```python
from build123d import *

# Parameters (mm, degrees)
SKETCH1_R           = 36.83
SKETCH1_R_2         = 24.13
SKETCH1_R_3         = 2.15265
BOSS_EXTRUDE1_DEPTH = 6.35


with BuildPart() as part:
    # Sketch1 → Boss-Extrude1 (new body)
    with BuildSketch(Plane(origin=(0, 0, 0), x_dir=(1, 0, 0), z_dir=(0, 1, 0))):
        Circle(SKETCH1_R)
        Circle(SKETCH1_R_2, mode=Mode.SUBTRACT)
        with Locations((0, 30.48)):
            Circle(SKETCH1_R_3, mode=Mode.SUBTRACT)
        with Locations((11.664191018, 28.159848151)):
            Circle(SKETCH1_R_3, mode=Mode.SUBTRACT)
        with Locations((21.552614691, 21.552614691)):
            Circle(SKETCH1_R_3, mode=Mode.SUBTRACT)
        with Locations((28.159848151, 11.664191018)):
            Circle(SKETCH1_R_3, mode=Mode.SUBTRACT)
        with Locations((30.48, 0)):
            Circle(SKETCH1_R_3, mode=Mode.SUBTRACT)
        with Locations((28.159848151, -11.664191018)):
            Circle(SKETCH1_R_3, mode=Mode.SUBTRACT)
        with Locations((21.552614691, -21.552614691)):
            Circle(SKETCH1_R_3, mode=Mode.SUBTRACT)
        with Locations((11.664191018, -28.159848151)):
            Circle(SKETCH1_R_3, mode=Mode.SUBTRACT)
        with Locations((0, -30.48)):
            Circle(SKETCH1_R_3, mode=Mode.SUBTRACT)
        with Locations((-11.664191018, -28.159848151)):
            Circle(SKETCH1_R_3, mode=Mode.SUBTRACT)
        with Locations((-21.552614691, -21.552614691)):
            Circle(SKETCH1_R_3, mode=Mode.SUBTRACT)
        with Locations((-28.159848151, -11.664191018)):
            Circle(SKETCH1_R_3, mode=Mode.SUBTRACT)
        with Locations((-30.48, 0)):
            Circle(SKETCH1_R_3, mode=Mode.SUBTRACT)
        with Locations((-28.159848151, 11.664191018)):
            Circle(SKETCH1_R_3, mode=Mode.SUBTRACT)
        with Locations((-21.552614691, 21.552614691)):
            Circle(SKETCH1_R_3, mode=Mode.SUBTRACT)
        with Locations((-11.664191018, 28.159848151)):
            Circle(SKETCH1_R_3, mode=Mode.SUBTRACT)
    extrude(amount=BOSS_EXTRUDE1_DEPTH)


solid = part.part
```
The listing builds one solid part. Answer for the finished solid, in the listing's coordinates (mm). Coordinates: 2 decimals unless noted, no trailing zeros. Write each loop counter-clockwise with the first axis right and the second up, starting at its lowest first coordinate (ties: lowest second). Pieces come first, ordered by that corner, then holes. Notation, with made-up numbers: (74.25, 52.5) - (125.25, 52.5) arc R31 cw to (125.25, 87.5) - close; hole circle Ø10 at (-17.5, 88). An arc over 180 degrees is marked (long way). Return JSON: item names as keys, results as strings. Group by question number.
Q1. Find the intervals of material crossed by line 1 along X through (y, z) = (1.75, 0); line 2 along Z through (x, y) = (28.5, 4); line 3 along Z through (x, y) = (-28, 0.75), in increasing order. Write a range as [from, to].
Q2. The part is cut by section D-D on z = -20.5. Write down the section's boundary in (x, y).
Q3. Flat-ended cylindrical pins translate along their axes: pin 1 Ø2.5 at (x, z) = (11.66, -28.16) entering from +Y; pin 2 Ø5 at (x, z) = (30.48, 0) entering from -Y; pin 3 Ø2 at (x, y) = (-18, 3.5) entering from +Z. Find the tip coordinate at first contact, or state that the pin passes through.
Q4. For a pull along Z with two mould halves and no side action, classify faces 1 (the cylindrical face through (-29.227, 3.131, 22.41)), 2 (the flat face through (-25, 0, -1)), 3 (the cylindrical face through (-29.87, 3.13, 12.97)) as +Z half, -Z half, draft (parallel to the pull), parting line (faces both ways), or undercut.
Q5. The part is cut by section B-B on x = -5.5. Write down the section's boundary in (y, z), and give its area (3 significant figures).
Q6. The part is cut by section C-C on y = 1. State how many separate pieces and enclosed holes the cut face has, and give its area (3 significant figures).
Q7. The part is cut by section A-A on z = 0. Write down the section's boundary in (x, y).
Evaluation:
{
 "1": {"line 1": "x = [-36.83, -32.63], [-28.33, -24.13], [24.13, 28.33], [32.63, 36.83]", "line 2": "z = [-23.33, -13.79], [-9.54, -0.84], [0.84, 9.54], [13.79, 23.33]", "line 3": "z = [-23.93, -13.81], [-9.52, 9.52], [13.81, 23.93]"},
 "2": {"outline": "(-30.6, 0) - (-23.43, 0) - (-23.43, 6.35) - (-30.6, 6.35) - close; (-19.67, 0) - (-12.73, 0) - (-12.73, 6.35) - (-19.67, 6.35) - close; (12.73, 0) - (19.67, 0) - (19.67, 6.35) - (12.73, 6.35) - close; (23.43, 0) - (30.6, 0) - (30.6, 6.35) - (23.43, 6.35) - close"},
 "3": {"pin 1": "passes through", "pin 2": "stops at y = 0", "pin 3": "stops at z = 32.67"},
 "4": {"face 1": "parting line", "face 2": "draft", "face 3": "undercut"},
 "5": {"outline": "(0, -36.42) - (6.35, -36.42) - (6.35, -23.49) - (0, -23.49) - close; (0, 23.49) - (6.35, 23.49) - (6.35, 36.42) - (0, 36.42) - close", "area": "164 mm2"},
 "6": {"separate pieces": "1", "enclosed holes": "17", "area": "2,200 mm2"},
 "7": {"outline": "(-36.83, 0) - (-32.63, 0) - (-32.63, 6.35) - (-36.83, 6.35) - close; (-28.33, 0) - (-24.13, 0) - (-24.13, 6.35) - (-28.33, 6.35) - close; (24.13, 0) - (28.33, 0) - (28.33, 6.35) - (24.13, 6.35) - close; (32.63, 0) - (36.83, 0) - (36.83, 6.35) - (32.63, 6.35) - close"}
}
